Autodesk Inventor part; units mm, degrees
ref_plane "bolt_XY" through (0, 0, 0) normal (1, 0, 0) x (0, 0, -1)
ref_plane "bolt_YZ" through (0, 0, 0) normal (0, 0, -1) x (0, 1, 0)
ref_plane "bolt_ZX" through (0, 0, 0) normal (0, 1, 0) x (1, 0, 0)
sketch "Sketch_8" plane through (0, 0, 0) normal (0, 0, 1) x (1, 0, 0)
  line L0 (35, 0) -> (-6, 0)
  line L1 (-6, 0) -> (-6, 4.5)
  line L2 (-6, 4.5) -> (-5.5, 5)
  line L3 (-5.5, 5) -> (0, 5)
  line L4 (0, 5) -> (0, 3.25)
  arc A0 (0, 3.25) -> (0.25, 3) centre (0.25, 3.25) ccw
  line L5 (0.25, 3) -> (34.3865, 3)
  line L6 (34.3865, 3) -> (35, 2.3865)
  line L7 (35, 2.3865) -> (35, 0)
  line L8 (35, 0) -> (-6, 0)
revolve "Revolution1" add sketch "Sketch_8" angle 360 about axis through (35, 0, 0) along (1, 0, 0)
thread "Thread1"
sketch "Sketch2" plane through (-6, 0, 0) normal (-1, 0, 0) x (0, 0, 1)
  point P0 (0, 0)
hole "Hole1" at (-6, 0, 0) direction (1, 0, 0) diameter 5 depth 3 tip angle 120
sketch "Sketch_3" plane through (-6, 0, 0) normal (1, 0, 0) x (0, 0, -1)
  line L0 (-2.5, -1.4434) -> (0, -2.8868)
  line L1 (0, -2.8868) -> (2.5, -1.4434)
  line L2 (2.5, -1.4434) -> (2.5, 1.4434)
  line L3 (2.5, 1.4434) -> (0, 2.8868)
  line L4 (0, 2.8868) -> (-2.5, 1.4434)
  line L5 (-2.5, 1.4434) -> (-2.5, -1.4434)
extrude "Extrusion1" cut sketch "Sketch_3" along normal blind 3
ref_plane "bolt_XY" through (0, 0, 0) normal (1, 0, 0) x (0, 0, -1)
ref_plane "bolt_YZ" through (0, 0, 0) normal (0, 0, -1) x (0, 1, 0)
ref_plane "bolt_ZX" through (0, 0, 0) normal (0, 1, 0) x (1, 0, 0)
ref_plane "nut_XY" through (35, 0, 0) normal (1, 0, 0) x (0, 0, -1)
ref_plane "nut_YZ" through (35, 0, 0) normal (0, 0, -1) x (0, 1, 0)
ref_plane "nut_ZX" through (35, 0, 0) normal (0, 1, 0) x (1, 0, 0)
properties part number "CBM6-35"
Geometry: final body of the model. Coordinates: model frame, mm. A direction names the side the tool comes from. Give positions to 0.01 mm unless a question says otherwise; leave off trailing zeros. Loops run counter-clockwise (first coordinate to the right, second up) from the corner with the lowest first, then second, coordinate; pieces in that order, holes last. Notation, with made-up numbers: M -27.5,65 L -17.5,65 A21 ccw -17.5,70 Z; hole C -39.75,-36.5 d10. An arc over 180 degrees is marked long. Put each result on its own line as item: value. Start each with the question number.
1) Access query for faces 5 (the flat face through (-4.521, -2.175, -1.233)), 6 (the flat face through (0, 3.3, -1)), 7 (the cylindrical face through (-2.71, -1.08, -4.88)). Directions: +Z, -Z, +X, -X, +Y, -Y. A direction counts if a zero-diameter tool reaches every point of the face in a straight line with its end or side. Return the directions, or none.
2) Cut plane A-A (x = 1). Output: boundary loops of the cut face in (y, z), then the cut area to 3 significant figures.
3) Ray query, line 1 along X through (y, z) = (-2.5, 3); line 2 along Z through (x, y) = (5.5, 0.75); line 3 along Z through (x, y) = (14.5, -0.25). Return the intervals inside material, ascending.
4) Contact query for flat-ended pins moving along their axis: pin 1 (1 mm diameter, centred on x = 22.5, z = -3, fed in from -Y); pin 2 (0.9 mm diameter, centred on x = -4.5, y = 0.5, fed in from -Z); pin 3 (2 mm diameter, centred on x = 8.5, y = 0, fed in from +Z); pin 4 (2.5 mm diameter, centred on y = 1, z = 0.5, fed in from -X). Output: stop coordinate, or through.
5) Pull-direction query (Y, two-part tool) for faces 1 (the flat face through (-5, 0, -2.5)), 2 (the flat face through (35, 0, 0)), 3 (the flat face through (-4.521, -2.155, 1.267)), 4 (the cylindrical face through (18, -3, 0)); classes: pulls with the +Y half, pulls with the -Y half, needs draft (parallel to the pull), parting line crosses it, or undercut.
Verdict:
1. face 5: -X
1. face 6: +X
1. face 7: +X, -X
2. outline: C 0,0 d6
2. area: 28.3 mm2
3. line 1: -6 to 0
3. line 2: -2.9 to 2.9
3. line 3: -2.99 to 2.99
4. pin 1: y = -1.66
4. pin 2: z = -5
4. pin 3: z = 3
4. pin 4: x = -2.92
5. face 1: undercut
5. face 2: needs draft
5. face 3: undercut
5. face 4: parting line crosses it
